Source: three-view drawing plus pictorial views. Frame: mm from the lowest corner of the part. A direction names the side the tool comes from. Give positions to 0.01 mm unless a question says otherwise; leave off trailing zeros. Loops run counter-clockwise (first coordinate to the right, second up) from the corner with the lowest first, then second, coordinate; pieces in that order, holes last.
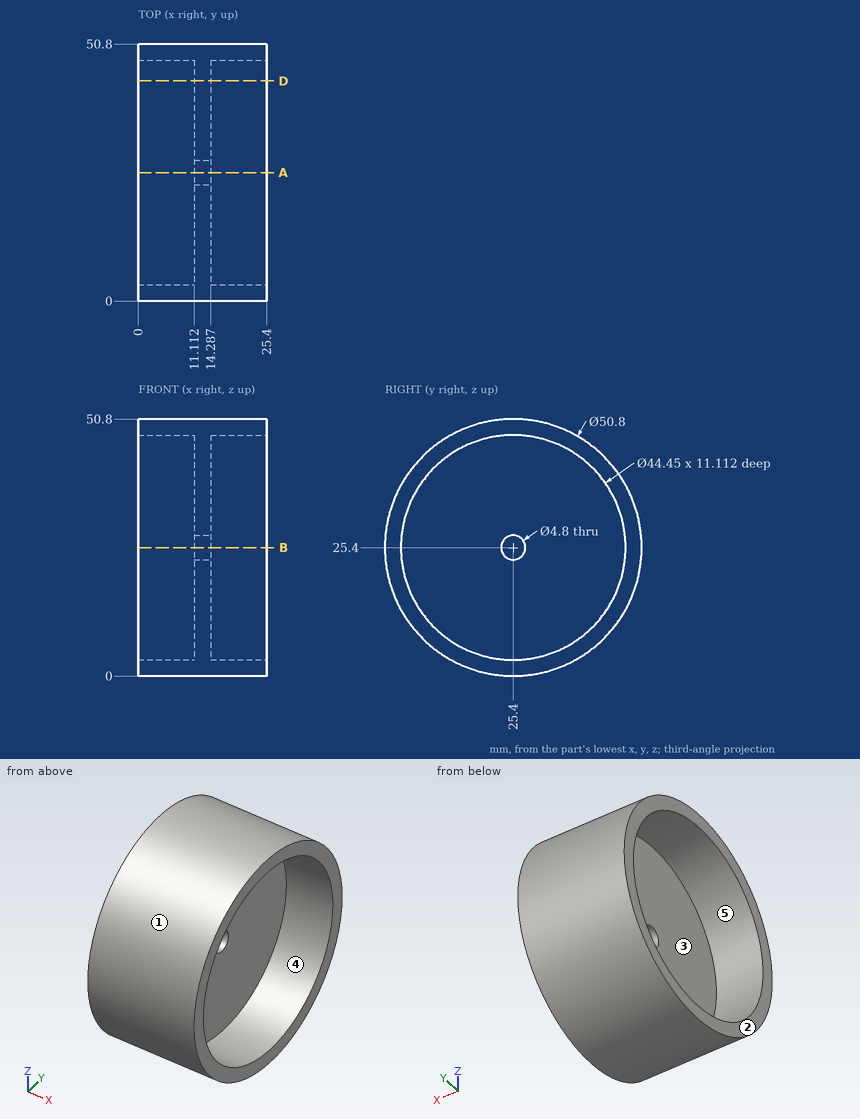
(1) Mould query, pull axis Z, two halves, no side actions, for the marked faces 1, 2 and 3. Classes: +Z half, -Z half, draft (parallel to the pull), parting line (faces both ways), or undercut.
Values follow:
face 1: parting line
face 2: draft
face 3: undercut
(2) Cut plane D-D (y = 43.5). Return the cut outline in (x, z), and give its area (3 significant figures).
Values follow:
outline: (0, 7.58) - (25.4, 7.58) - (25.4, 12.5) - (14.29, 12.5) - (14.29, 38.3) - (25.4, 38.3) - (25.4, 43.22) - (0, 43.22) - (0, 38.3) - (11.11, 38.3) - (11.11, 12.5) - (0, 12.5) - close
area: 332 mm2
(3) Ray query, probe 1 along Z at (x, y) = (19.5, 25.4) (1 decimal); probe 2 along X at (y, z) = (38.5, 7.5); probe 3 along Z at (x, y) = (16, 16) (1 decimal). Return the intervals inside material, ascending.
Values follow:
probe 1: z = 0 to 3.2, 47.6 to 50.8
probe 2: x = 11.11 to 14.29
probe 3: z = 1.8 to 5.3, 45.5 to 49
(4) Pin query (flat end, axial travel): pin 1 Ø13.5 at (y, z) = (15, 27.5) entering from -X; pin 2 Ø4.5 at (y, z) = (25.4, 25.4) entering from -X; pin 3 Ø1 at (x, y) = (7.5, 13) entering from +Z; pin 4 Ø5 at (x, z) = (23, 45.5) entering from +Y (1 decimal). Return the tip coordinate at first contact, or that it passes through.
Values follow:
pin 1: stops at x = 11.11
pin 2: passes through
pin 3: stops at z = 47.84
pin 4: stops at y = 43.7
(5) Reachability of the marked faces 4 and 5 from +Z, -Z, +X, -X, +Y, -Y: full face, straight path, thin tool, end or side. Return the list, or none.
Values follow:
face 4: +X
face 5: -X
(6) Cut plane A-A (y = 25.4). Return the cut outline in (x, z) (1 decimal).
Values follow:
outline: (0, 0) - (25.4, 0) - (25.4, 3.2) - (14.3, 3.2) - (14.3, 23) - (11.1, 23) - (11.1, 3.2) - (0, 3.2) - close; (0, 47.6) - (11.1, 47.6) - (11.1, 27.8) - (14.3, 27.8) - (14.3, 47.6) - (25.4, 47.6) - (25.4, 50.8) - (0, 50.8) - close
